Read the model definition and answer for the solid it produces. Units are mm, in the model's axes. A direction names the side the tool comes from. Give positions to 0.01 mm unless a question says otherwise; leave off trailing zeros. Write each loop counter-clockwise with the first axis right and the second up, starting at its lowest first coordinate (ties: lowest second). Pieces come first, ordered by that corner, then holes. Notation, with made-up numbers: M 7,51.25 L 61,51.25 A31 ccw 61,78.25 Z; hole C 10.5,-31.5 d11. An arc over 180 degrees is marked long. Put each result on its own line as item: value.
from build123d import *

# Parameters (mm, degrees)
F0_W        = 203.2
F0_H        = 127
F1_DEPTH    = 127
F3_DEPTH    = 76.2
F4_SIZE2    = 101.6
F4_SIZE     = 76.2
F5_R        = 5.08
F6_T1_DEPTH = 76.2
F6_T3_DEPTH = 134.62
F6_S7_W     = 5.08
F6_S7_H     = 5.08
F6_T8_DEPTH = 5.08
F7_R        = 15.24
F8_DEPTH    = 50.8
F9_R        = 19.05
F10_DEPTH   = 127


# Not quite as in the source:
# - a fillet or chamfer that OpenCascade refuses, or shapes differently, is made with other operations: its cross-section is extruded or revolved along the edge and cut away or added


with BuildPart() as f1:
    # F0 (on Front) → F1 (new body)
    with BuildSketch(Plane.XZ):
        with Locations((12.863317194, -0.4497872638)):
            Rectangle(F0_W, F0_H)
    extrude(amount=F1_DEPTH)

    # F2 (on face) → F3 (cut)
    with BuildSketch(Plane.XZ.offset(127)):
        Polygon((114.463317194, 63.0502127362), (12.863317194, 63.0502127362), (12.863317194, -0.4497872638), (-25.236682806, -0.4497872638), (-25.236682806, -63.9497872638), (114.463317194, -63.9497872638), align=None)
    extrude(amount=-F3_DEPTH, mode=Mode.SUBTRACT)

    # F4
    f4_edges = [f1.edges().sort_by_distance(p)[0] for p in [
        (114.463317, -25.4, 63.050213),
    ]]
    f4_side = f1.faces().sort_by_distance((-8.908111, -52.614286, 63.050213))[0]
    chamfer(f4_edges, length=F4_SIZE, length2=F4_SIZE2, reference=f4_side)

    # F5
    f5_edges = [f1.edges().sort_by_distance(p)[0] for p in [
        (-37.936683, -127, 63.050213),
        (-88.736683, -63.5, 63.050213),
        (12.863317, -88.9, 63.050213),
        (25.563317, -50.8, 63.050213),
        (-25.236683, 0, 63.050213),
    ]]
    fillet(f5_edges, radius=F5_R)

    # F6: fillet of radius 5.08 on 2 edges, made by hand

    # F6_s2 → F6_t1 (cut)
    with BuildSketch(Plane.XY.offset(-76.6497872638)):
        with BuildLine():
            ThreePointArc((-30.316682806, -127), (-26.7245803576, -125.5121024484), (-25.236682806, -121.92))
            Line((-25.236682806, -121.92), (-25.236682806, -127))
            Line((-25.236682806, -127), (-30.316682806, -127))
        make_face()
    extrude(amount=F6_T1_DEPTH, mode=Mode.SUBTRACT)

    # F6_s4 → F6_t3 (cut)
    with BuildSketch(Plane.XY.offset(-76.6497872638)):
        with BuildLine():
            ThreePointArc((-88.736682806, -121.92), (-87.2487852545, -125.5121024484), (-83.656682806, -127))
            Line((-83.656682806, -127), (-88.736682806, -127))
            Line((-88.736682806, -127), (-88.736682806, -121.92))
        make_face()
    extrude(amount=F6_T3_DEPTH, mode=Mode.SUBTRACT)


with BuildPart() as f6_tool6:
    # F6_s7 → F6_t8 (new body)
    with BuildSketch(Plane.YZ.offset(-83.656682806)):
        with Locations((-124.46, 60.5102127362)):
            Rectangle(F6_S7_W, F6_S7_H)
    extrude(amount=-F6_T8_DEPTH)

    # F6_s9 → F6_t10 (revolve, cut)
    with BuildSketch(Plane(origin=(-83.656682806, -121.92, 57.9702127362), x_dir=(0, 0.7071067812, -0.7071067812), z_dir=(0, 0.7071067812, 0.7071067812))):
        with BuildLine():
            ThreePointArc((0, -5.08), (5.08, 0), (0, 5.08))
            Line((0, 5.08), (0, -5.08))
        make_face()
    revolve(axis=Axis((-83.656682806, -121.92, 57.9702127362), (-1, 0, 0)), mode=Mode.SUBTRACT)


with BuildPart() as f1_1:
    add(f1.part)

    # F6_t5: cut F6_tool6
    add(f6_tool6.part, mode=Mode.SUBTRACT)

    # F7 (on face) → F8 (cut, through all)
    with BuildSketch(Plane.XZ.offset(50.8)):
        with Locations((37.6529693604, -29.2071215808)):
            Circle(F7_R)
    extrude(amount=-F8_DEPTH, mode=Mode.SUBTRACT)

    # F9 (on face) → F10 (cut, through all)
    with BuildSketch(Plane.XY.offset(63.0502127362)):
        with Locations((-53.0607067049, -93.1101441383)):
            Circle(F9_R)
    extrude(amount=-F10_DEPTH, mode=Mode.SUBTRACT)


solid = f1_1.part
(1) Section C-C on y = -90.5 is taken. Determine the outline of the cut face in (x, z).
Result:
outline: M -88.74,-63.95 L -71.93,-63.95 L -71.93,63.05 L -83.66,63.05 A5.08 ccw -88.74,57.97 Z; M -34.19,-63.95 L -25.24,-63.95 L -25.24,-0.45 L 12.86,-0.45 L 12.86,57.97 A5.08 ccw 7.78,63.05 L -34.19,63.05 Z
(2) Straight lines are drawn through the part: line 1 along Y through (x, z) = (-38, -46.5); line 2 along Y through (x, z) = (-36.5, -13); line 3 along Z through (x, y) = (50.5, -14.5). For each, find the intervals that lie inside material, in ascending order. Write a range as from..to.
Result:
line 1: y = -127..-104.78, -81.44..0
line 2: y = -127..-102.53, -83.69..0
line 3: z = -63.95..-37.41, -21.01..46.73
(3) Given pin 1 Ø12 at (y, z) = (-66, -17.5) entering from +X; pin 2 Ø1.5 at (x, z) = (53, -18.5) entering from -Y; pin 3 Ø17.5 at (y, z) = (-75.5, 29) entering from +X, each flat-ended and moving along its own axis, determine where each tip first touches the part or whether it passes through.
Result:
pin 1: stops at x = -25.24
pin 2: stops at y = -50.8
pin 3: stops at x = 12.86
(4) Section A-A on z = -32 is taken. Determine the outline of the cut face in (x, y), and give its area (3 significant figures).
Result:
outline: M -88.74,-121.92 A5.08 ccw -83.66,-127 L -30.32,-127 A5.08 ccw -25.24,-121.92 L -25.24,-50.8 L 22.67,-50.8 L 22.67,0 L -88.74,0 Z; M 52.63,-50.8 L 109.55,-50.8 L 109.55,0 L 52.63,0 Z; hole C -53.06,-93.11 d38.1
area: 12,200 mm²
(5) Section D-D on z = 14 is taken. Determine the outline of the cut face in (x, y).
Result:
outline: M -88.74,-121.92 A5.08 ccw -83.66,-127 L 12.86,-127 L 12.86,-50.8 L 75.05,-50.8 L 75.05,0 L -88.74,0 Z; hole C -53.06,-93.11 d38.1
(6) Which of the six approach directions +Z, -Z, +X, -X, +Y, -Y give full straight-line access (tool end or side, diameter ignored) to faces 1 (the face through (24.688, -49.272, 61.602)), 2 (the face through (-4, -89, -0.45)), 3 (the face through (-22.416, -1.528, 61.602))?
Result:
face 1: +Z, +X, -Y
face 2: -Z, +X, -Y
face 3: +Z, +X, -X, +Y
(7) For a pull along X with two mould halves and no side action, classify faces 4 (the face through (-24, -50, 63.05)), 5 (the face through (-55.541, -74.222, 0.439)), 6 (the face through (12.863, -89, 29)) as +X half, -X half, draft (parallel to the pull), parting line (faces both ways), or undercut.
Result:
face 4: draft
face 5: undercut
face 6: +X half
(8) Section B-B on x = 49.5 is taken. Determine the outline of the cut face in (y, z).
Result:
outline: M -50.8,-63.95 L 0,-63.95 L 0,-38.79 L -50.8,-38.79 Z; M -50.8,-19.62 L 0,-19.62 L 0,48.07 L -50.8,48.07 Z
